Work out the finished part from the listing and answer in its coordinate system (mm). A direction names the side the tool comes from. Give positions to 0.01 mm unless a question says otherwise; leave off trailing zeros. Loops run counter-clockwise (first coordinate to the right, second up) from the corner with the lowest first, then second, coordinate; pieces in that order, holes last. Notation, with made-up numbers: M 64.25,-20.75 L 122.25,-20.75 A14 ccw 122.25,-15.75 Z; hole C 33,70 d3. An arc over 180 degrees is marked long. Answer in a Markdown table with one row per item. Add a question column.
from build123d import *

# Parameters (mm, degrees)
SKETCH1_W           = 266.7
SKETCH1_H           = 247.65
BOSS_EXTRUDE1_DEPTH = 6.35
SKETCH2_W           = 247.65
SKETCH2_H           = 95.758
BOSS_EXTRUDE2_DEPTH = 12.7
SKETCH3_W           = 292.1
SKETCH3_H           = 95.758
BOSS_EXTRUDE3_DEPTH = 12.7
SKETCH4_W           = 19.05
SKETCH4_H           = 247.65
BOSS_EXTRUDE4_DEPTH = 0.762
FILLET1_R           = 5.08
SKETCH6_W           = 281.94
SKETCH6_H           = 12.7
BOSS_EXTRUDE5_DEPTH = 25.4
FILLET2_R           = 12.7


with BuildPart() as part:
    # Sketch1 → Boss-Extrude1 (new body)
    with BuildSketch(Plane(origin=(0, 0, 0), x_dir=(1, 0, 0), z_dir=(0, 1, 0))):
        Rectangle(SKETCH1_W, SKETCH1_H)
    extrude(amount=BOSS_EXTRUDE1_DEPTH)

    # Sketch2 → Boss-Extrude2 (add)
    with BuildSketch(Plane.ZY.offset(133.35)):
        with Locations((0, 47.879)):
            Rectangle(SKETCH2_W, SKETCH2_H)
    boss_extrude2 = extrude(amount=BOSS_EXTRUDE2_DEPTH)

    # Mirror1: Boss-Extrude2 across plane
    add(boss_extrude2.mirror(Plane(origin=(0, 0, 0), x_dir=(0, 0, 1), z_dir=(1, 0, 0))))

    # Sketch3 → Boss-Extrude3 (add)
    with BuildSketch(Plane(origin=(0, 0, -123.825), x_dir=(-1, 0, 0), z_dir=(0, 0, -1))):
        with Locations((0, 47.879)):
            Rectangle(SKETCH3_W, SKETCH3_H)
    extrude(amount=BOSS_EXTRUDE3_DEPTH)

    # Sketch4 → Boss-Extrude4 (add)
    with BuildSketch(Plane(origin=(0, 6.35, 0), x_dir=(1, 0, 0), z_dir=(0, 1, 0))):
        with Locations((-107.95, 0)):
            Rectangle(SKETCH4_W, SKETCH4_H)
        with Locations((-69.85, 0)):
            Rectangle(SKETCH4_W, SKETCH4_H)
        with Locations((-19.05, 0)):
            Rectangle(SKETCH4_W, SKETCH4_H)
        with Locations((19.05, 0)):
            Rectangle(SKETCH4_W, SKETCH4_H)
        with Locations((69.85, 0)):
            Rectangle(SKETCH4_W, SKETCH4_H)
        with Locations((107.95, 0)):
            Rectangle(SKETCH4_W, SKETCH4_H)
    extrude(amount=BOSS_EXTRUDE4_DEPTH)

    # Fillet1
    fillet1_edges = [part.edges().sort_by_distance(p)[0] for p in [
        (-146.05, 0, -6.35),
        (-146.05, 47.879, 123.825),
        (-146.05, 95.758, -6.35),
        (146.05, 0, -6.35),
        (146.05, 95.758, -6.35),
        (146.05, 47.879, 123.825),
        (0, 0, -136.525),
        (-146.05, 47.879, -136.525),
        (0, 95.758, -136.525),
        (146.05, 47.879, -136.525),
    ]]
    fillet(fillet1_edges, radius=FILLET1_R)

    # Sketch6 → Boss-Extrude5 (add)
    with BuildSketch(Plane.XY.offset(123.825)):
        with Locations((0, 102.108)):
            Rectangle(SKETCH6_W, SKETCH6_H)
    extrude(amount=-BOSS_EXTRUDE5_DEPTH)

    # Fillet2
    fillet2_edges = [part.edges().sort_by_distance(p)[0] for p in [
        (140.97, 108.458, 111.125),
        (-140.97, 108.458, 111.125),
    ]]
    fillet(fillet2_edges, radius=FILLET2_R - 0.0001)  # a hair under: the kernel refuses the full size


solid = part.part
(1) Section C-C, the plane x = 102 is taken. Determine the outline of the cut face in (y, z) (3 decimals), and give its area (3 significant figures).
(2) Consider line 1 along X through (y, z) = (56, -123); line 2 along Y through (x, z) = (-94.5, 109). Determine where each line is inside the solid, lowest interval first. Write a range as from..to.
(3) Which of the six approach directions +Z, -Z, +X, -X, +Y, -Y give full straight-line access (tool end or side, diameter ignored) to faces 5 (the face through (-2, 95.758, 111)), 6 (the face through (2, 0, -2)), 7 (the face through (-2, 102, 98.425))?
(4) Section A-A, the plane x = 4.5 is taken. Determine the outline of the cut face in (y, z) (3 decimals).
(5) The mould has two halves that part along X. Classify faces 1 (the face through (-45, 6.35, -2)), 2 (the face through (137.15, 104.84, 110.95)), 3 (the face through (1, 95.758, -127)), 4 (the face through (108, 7.112, -2)): pulls with the +X half, pulls with the -X half, needs draft (parallel to the pull), parting line crosses it, or undercut.
(6) Section B-B, the plane y = 35.5 is taken. Determine the outline of the cut face in (x, z) (3 decimals), and give its area (3 significant figures).
(7) Each of these flat-tipped pins is pushed along its axis until it touches: P1, Ø2, axis at x = 71.5, z = -22.5, coming from the +Y side; P2, Ø4, axis at x = -55.5, z = -31.5, coming from the +Y side; P3, Ø4, axis at x = -1.5, y = 104.5, coming from the -Z side (3 decimals). Where does it stop, or does it pass through?
Numbers:
| question | item | result |
|---|---|---|
| 1 | outline | M 0,-131.445 A5.08 ccw 5.08,-136.525 L 90.678,-136.525 A5.08 ccw 95.758,-131.445 L 95.758,-123.825 L 7.112,-123.825 L 7.112,123.825 L 0,123.825 Z; M 95.758,98.425 L 108.458,98.425 L 108.458,123.825 L 95.758,123.825 Z |
| 1 | area | 3,290 mm² |
| 2 | line 1 | x = -146.05..-133.35, 133.35..146.05 |
| 2 | line 2 | y = 0..6.35, 95.76..108.46 |
| 3 | face 5 | +Z |
| 3 | face 6 | +Z, -Z, +X, -X, -Y |
| 3 | face 7 | -Z, +X, -X, +Y |
| 4 | outline | M 0,-131.445 A5.08 ccw 5.08,-136.525 L 90.678,-136.525 A5.08 ccw 95.758,-131.445 L 95.758,-123.825 L 6.35,-123.825 L 6.35,123.825 L 0,123.825 Z; M 95.758,98.425 L 108.458,98.425 L 108.458,123.825 L 95.758,123.825 Z |
| 5 | face 1 | undercut |
| 5 | face 2 | pulls with the +X half |
| 5 | face 3 | needs draft |
| 5 | face 4 | undercut |
| 6 | outline | M -146.05,-131.445 A5.08 ccw -140.97,-136.525 L 140.97,-136.525 A5.08 ccw 146.05,-131.445 L 146.05,118.745 A5.08 ccw 140.97,123.825 L 133.35,123.825 L 133.35,-123.825 L -133.35,-123.825 L -133.35,123.825 L -140.97,123.825 A5.08 ccw -146.05,118.745 Z |
| 6 | area | 9,980 mm² |
| 7 | P1 | stops at y = 7.11 |
| 7 | P2 | stops at y = 6.35 |
| 7 | P3 | stops at z = 98.425 |
